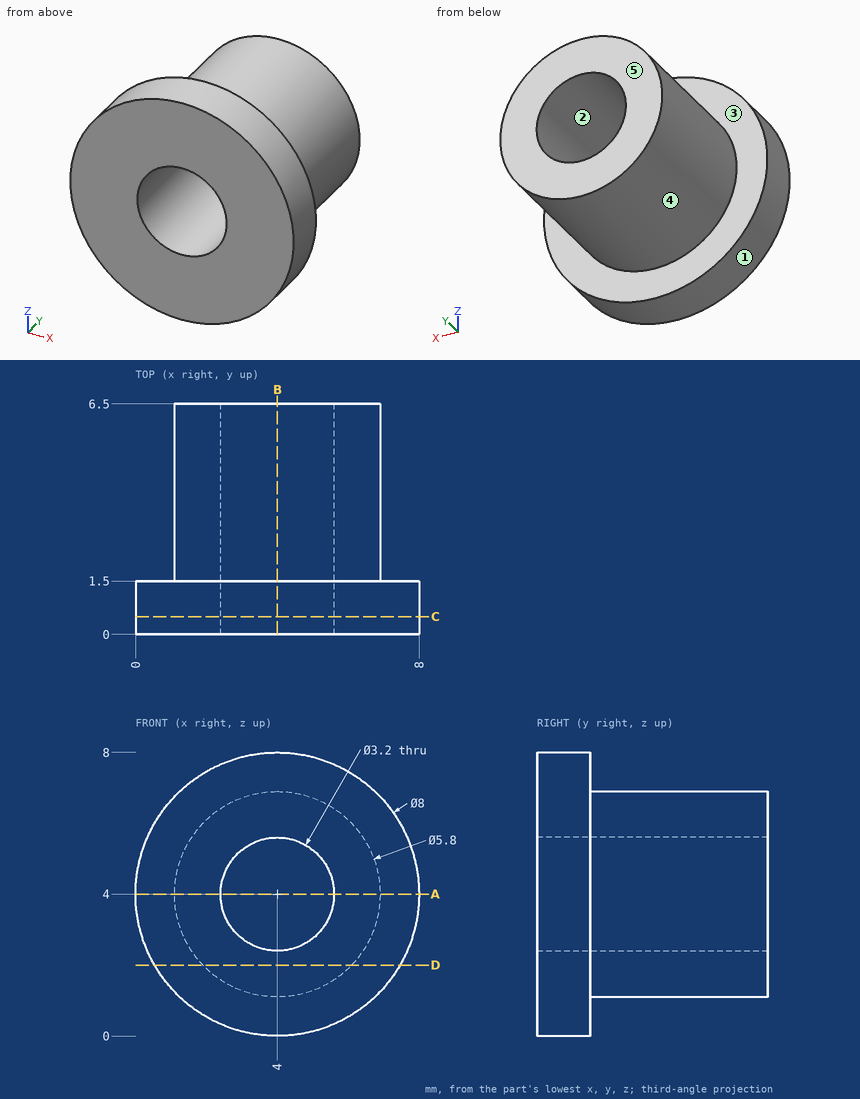
Answer from the drawing. Dimensions are ordinates in mm from the lowest x, y and z of the part. A direction names the side the tool comes from. Round coordinates to 2 decimals unless told otherwise and drop trailing zeros. Write each loop counter-clockwise with the first axis right and the second up, starting at its lowest first coordinate (ties: lowest second). Pieces come first, ordered by that corner, then holes. Notation, with made-up numbers: M -36.5,83 L -31.5,83 A11 ccw -31.5,92 Z; hole C 88,47.25 d10. An arc over 180 degrees is marked long. Write each question's results on one line, items separated by ' | '. Start each with the question number.
Item 1: Which of the six approach directions +Z, -Z, +X, -X, +Y, -Y give full straight-line access (tool end or side, diameter ignored) to the marked faces 4 and 5?
Item 2: Find section C-C on y = 0.5. Write down the section's boundary in (x, z), and give its area (3 significant figures).
Item 3: Find section D-D on z = 2. Write down the section's boundary in (x, y), and give its area (3 significant figures).
Item 4: Given pin 1 Ø2 at (x, y) = (6.5, 2) entering from +Z; pin 2 Ø2 at (x, y) = (6.5, 5.5) entering from -Z, each flat-ended and moving along its own axis, determine where each tip first touches the part or whether it passes through.
Item 5: The mould has two halves that part along X. Classify the marked faces 1, 2 and 3: +X half, -X half, draft (parallel to the pull), parting line (faces both ways), or undercut.
Item 6: Find section A-A on z = 4. Write down the section's boundary in (x, y), and give its area (3 significant figures).
Item 7: Straight lines are drawn through the part: probe 1 along X at (y, z) = (3.5, 4); probe 2 along X at (y, z) = (0.75, 4); probe 3 along Z at (x, y) = (3.25, 0.75). For each, find the intervals that lie inside material, in ascending order.
Item 8: Find section B-B on x = 4. Write down the section's boundary in (y, z), and give its area (3 significant figures).
Answer block:
1) face 4: +Y | face 5: +Z, -Z, +X, -X, +Y
2) outline: C 4,4 d8; hole C 4,4 d3.2 | area: 42.2 mm²
3) outline: M 0.54,0 L 7.46,0 L 7.46,1.5 L 6.1,1.5 L 6.1,6.5 L 1.9,6.5 L 1.9,1.5 L 0.54,1.5 Z | area: 31.4 mm²
4) pin 1: stops at z = 7.65 | pin 2: stops at z = 1.52
5) face 1: parting line | face 2: undercut | face 3: draft
6) outline: M 0,0 L 2.4,0 L 2.4,6.5 L 1.1,6.5 L 1.1,1.5 L 0,1.5 Z; M 5.6,0 L 8,0 L 8,1.5 L 6.9,1.5 L 6.9,6.5 L 5.6,6.5 Z | area: 20.2 mm²
7) probe 1: x = 1.1 to 2.4, 5.6 to 6.9 | probe 2: x = 0 to 2.4, 5.6 to 8 | probe 3: z = 0.07 to 2.59, 5.41 to 7.93
8) outline: M 0,0 L 1.5,0 L 1.5,1.1 L 6.5,1.1 L 6.5,2.4 L 0,2.4 Z; M 0,5.6 L 6.5,5.6 L 6.5,6.9 L 1.5,6.9 L 1.5,8 L 0,8 Z | area: 20.2 mm²
